Could you check a few things on this model? Use its own coordinates, in mm. A direction names the side the tool comes from. Give positions to 0.01 mm unless a question says otherwise; leave off trailing zeros. Order: outer loops, then holes, each group sorted by start corner. A loop starts at its lowest first (then second) coordinate and runs counter-clockwise, first axis right, second up. Notation, with made-up numbers: M -17.75,17.5 L 20.25,17.5 A11 cw 20.25,32.5 Z; hole C 17.5,58.5 d2. An arc over 180 degrees is marked long. Answer in a Markdown table with one row per item. Add a question column.
```python
from build123d import *

# Parameters (mm, degrees)
F0_W     = 406.4
F0_H     = 88.9
F1_DEPTH = 6.35
F2_W     = 6.35
F2_H     = 88.9
F3_DEPTH = 88.9
F5_DEPTH = 25.4


with BuildPart() as f1:
    # F0 (on Front) → F1 (new body)
    with BuildSketch(Plane.XZ):
        with Locations((151.11976, 18.916855)):
            Rectangle(F0_W, F0_H)
    extrude(amount=F1_DEPTH)

    # F2 (on face) → F3 (join)
    with BuildSketch(Plane.XZ.offset(6.35)):
        with Locations((-48.90524, 18.916855)):
            Rectangle(F2_W, F2_H)
    extrude(amount=F3_DEPTH)

    # F4 (on face) → F5 (cut)
    with BuildSketch(Plane(origin=(-52.08024, 0, 0), x_dir=(0, -1, 0), z_dir=(-1, 0, 0))):
        with BuildLine():
            Line((17.78, 35.426855), (17.78, 45.586855))
            ThreePointArc((17.78, 45.586855), (14.187898, 44.098957), (12.7, 40.506855))
            ThreePointArc((12.7, 40.506855), (14.187898, 36.914752), (17.78, 35.426855))
        make_face()
        with BuildLine():
            ThreePointArc((22.86, 40.506855), (21.372102, 44.098957), (17.78, 45.586855))
            Line((17.78, 45.586855), (17.78, 35.426855))
            ThreePointArc((17.78, 35.426855), (21.372102, 36.914752), (22.86, 40.506855))
        make_face()
        with BuildLine():
            ThreePointArc((12.7, -2.673145), (14.187898, -6.265248), (17.78, -7.753145))
            Line((17.78, -7.753145), (17.78, 2.406855))
            ThreePointArc((17.78, 2.406855), (14.187898, 0.918957), (12.7, -2.673145))
        make_face()
        with BuildLine():
            Line((17.78, 2.406855), (17.78, -7.753145))
            ThreePointArc((17.78, -7.753145), (21.372102, -6.265248), (22.86, -2.673145))
            ThreePointArc((22.86, -2.673145), (21.372102, 0.918957), (17.78, 2.406855))
        make_face()
        with BuildLine():
            ThreePointArc((83.82, 35.426855), (78.74, 40.506855), (83.82, 45.586855))
            Line((83.82, 45.586855), (17.78, 45.586855))
            ThreePointArc((17.78, 45.586855), (21.372102, 44.098957), (22.86, 40.506855))
            ThreePointArc((22.86, 40.506855), (21.372102, 36.914752), (17.78, 35.426855))
            Line((17.78, 35.426855), (83.82, 35.426855))
        make_face()
        with BuildLine():
            Line((83.82, 35.426855), (83.82, 45.586855))
            ThreePointArc((83.82, 45.586855), (78.74, 40.506855), (83.82, 35.426855))
        make_face()
        with BuildLine():
            ThreePointArc((83.82, 35.426855), (87.412102, 36.914752), (88.9, 40.506855))
            ThreePointArc((88.9, 40.506855), (87.412102, 44.098957), (83.82, 45.586855))
            Line((83.82, 45.586855), (83.82, 35.426855))
        make_face()
        with BuildLine():
            Line((17.78, -7.753145), (83.82, -7.753145))
            ThreePointArc((83.82, -7.753145), (78.74, -2.673145), (83.82, 2.406855))
            Line((83.82, 2.406855), (17.78, 2.406855))
            ThreePointArc((17.78, 2.406855), (21.372102, 0.918957), (22.86, -2.673145))
            ThreePointArc((22.86, -2.673145), (21.372102, -6.265248), (17.78, -7.753145))
        make_face()
        with BuildLine():
            ThreePointArc((83.82, 2.406855), (78.74, -2.673145), (83.82, -7.753145))
            Line((83.82, -7.753145), (83.82, 2.406855))
        make_face()
        with BuildLine():
            ThreePointArc((83.82, -7.753145), (87.412102, -6.265248), (88.9, -2.673145))
            ThreePointArc((88.9, -2.673145), (87.412102, 0.918957), (83.82, 2.406855))
            Line((83.82, 2.406855), (83.82, -7.753145))
        make_face()
    extrude(amount=-F5_DEPTH, mode=Mode.SUBTRACT)


solid = f1.part
```
1. If I drill on line 1 along Y through (x, z) = (-34, -20.5); line 2 along X through (y, z) = (-69, 56), over which ranges is the centre line in solid material (lowest first)? Write a range as [from, to].
2. Suppose I cut it at B-B on z = 12.5. List the corners of the cut face in (x, y) for me, plus the area to 3 significant figures.
3. Suppose I cut it at A-A on y = -48. List the corners of the cut face in (x, z) for me.
4. For faces 1 (the flat face through (150, -2, 63.367)), 2 (the flat face through (151, -6.35, 20)), which set-ups out of +Z, -Z, +X, -X, +Y, -Y let a thin tool reach every point of the face, with its end or its side?
5. Suppose I cut it at C-C on x = 184. List the corners of the cut face in (y, z) for me, plus the area to 3 significant figures.
6. Will these pins go through, and if not, where does the flat tip stop? P1, Ø12, axis at x = -10, z = 10, coming from the -Y side; P2, Ø1.5, axis at y = -34, z = 52.5, coming from the +X side.
Findings below:
| question | item | result |
|---|---|---|
| 1 | line 1 | [-6.35, 0] |
| 1 | line 2 | [-52.08, -45.73] |
| 2 | outline | M -52.08,-95.25 L -45.73,-95.25 L -45.73,-6.35 L 354.32,-6.35 L 354.32,0 L -52.08,0 Z |
| 2 | area | 3,150 mm2 |
| 3 | outline | M -52.08,-25.53 L -45.73,-25.53 L -45.73,-7.75 L -52.08,-7.75 Z; M -52.08,2.41 L -45.73,2.41 L -45.73,35.43 L -52.08,35.43 Z; M -52.08,45.59 L -45.73,45.59 L -45.73,63.37 L -52.08,63.37 Z |
| 4 | face 1 | +Z, +X, -X, +Y, -Y |
| 4 | face 2 | +Z, -Z, +X, -Y |
| 5 | outline | M -6.35,-25.53 L 0,-25.53 L 0,63.37 L -6.35,63.37 Z |
| 5 | area | 565 mm2 |
| 6 | P1 | y = -6.35 |
| 6 | P2 | x = -45.73 |
